Verification items for this drawing (mm, ordinates from the low corner). A direction names the side the tool comes from. Give positions to 0.01 mm unless a question says otherwise; leave off trailing zeros. Write each loop counter-clockwise with the first axis right and the second up, starting at its lowest first coordinate (ties: lowest second). Pieces come first, ordered by that corner, then holes. Notation, with made-up numbers: M 18.25,-34.75 L 28.25,-34.75 A15 cw 28.25,-13.75 Z; hole C -20,16.25 d4. An arc over 180 degrees is marked long. Use one line per item in the form item = value. Start each with the question number.
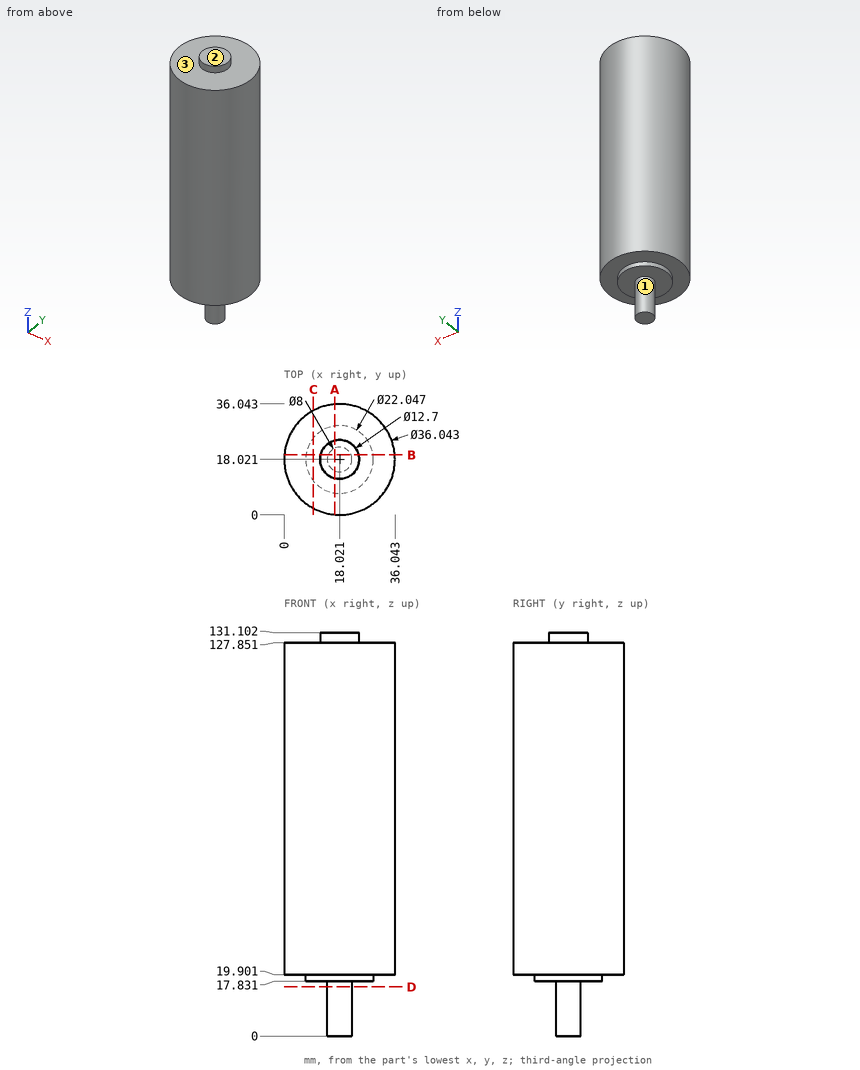
(1) Sectioned sample at B-B, the plane y = 19.5. Record the boundary of the cut face in (x, z) (1 decimal).
(2) Sectioned sample at D-D, the plane z = 16. Record the boundary of the cut face in (x, y).
(3) Sectioned sample at A-A, the plane x = 16.5. Record the boundary of the cut face in (y, z) (1 decimal), plus the area to 3 significant figures.
(4) Tool access check on the marked faces 1, 2 and 3. Record the directions out of +Z, -Z, +X, -X, +Y, -Y that give a thin tool (end or side, any length) a straight path to the whole face; none if there is none.
(5) Depth check by flat-ended pin: pin 1 (1.5 mm diameter, centred on x = 13, z = 90, fed in from +Y); pin 2 (8 mm diameter, centred on y = 28, z = 72, fed in from +X); pin 3 (6 mm diameter, centred on x = 32, z = 85.5, fed in from +Y); pin 4 (17.5 mm diameter, centred on x = 13.5, y = 19.5, fed in from -Z). Enter the tip coordinate at first touch or a pass-through.
(6) Thickness scan on probe 1 along Z at (x, y) = (13, 3); probe 2 along Z at (x, y) = (23.5, 20); probe 3 along X at (y, z) = (17.5, 126) (1 decimal). Record the ranges inside material, lowest first. Write a range as [from, to].
(7) Sectioned sample at C-C, the plane x = 9.5. Record the boundary of the cut face in (y, z) (1 decimal).
Numbers:
q1.outline = M 0.1,19.9 L 7.1,19.9 L 7.1,17.8 L 14.3,17.8 L 14.3,0 L 21.7,0 L 21.7,17.8 L 28.9,17.8 L 28.9,19.9 L 36,19.9 L 36,127.9 L 24.2,127.9 L 24.2,131.1 L 11.8,131.1 L 11.8,127.9 L 0.1,127.9 Z
q2.outline = C 18.02,18.02 d8
q3.outline = M 0.1,19.9 L 7.1,19.9 L 7.1,17.8 L 14.3,17.8 L 14.3,0 L 21.7,0 L 21.7,17.8 L 28.9,17.8 L 28.9,19.9 L 36,19.9 L 36,127.9 L 24.2,127.9 L 24.2,131.1 L 11.9,131.1 L 11.9,127.9 L 0.1,127.9 Z
q3.area = 4,090 mm2
q4.face_1 = -Z
q4.face_2 = +Z, +X, -X, +Y, -Y
q4.face_3 = +Z
q5.pin_1 = 35.53
q5.pin_2 = 35.02
q5.pin_3 = 32.31
q5.pin_4 = 0
q6.probe_1 = [19.9, 127.85]
q6.probe_2 = [17.83, 131.1]
q6.probe_3 = [0, 36]
q7.outline = M 2.1,19.9 L 11,19.9 L 11,17.8 L 25,17.8 L 25,19.9 L 33.9,19.9 L 33.9,127.9 L 2.1,127.9 Z
